The drawing under review shows one solid part. Ordinate dimensions are in mm from its lowest x, y, z. Round coordinates to 2 decimals unless told otherwise and drop trailing zeros. Write each loop counter-clockwise with the first axis right and the second up, starting at its lowest first coordinate (ties: lowest second). Pieces come first, ordered by that corner, then holes. Notation, with made-up numbers: (42.25, 70) -> (61.25, 70) arc R15 ccw to (61.25, 84) -> close; hole circle Ø4 at (73.5, 18.25). An arc over 180 degrees is marked (long way). Use CSV: the item, a comma, the result in double quotes. Start each with the question number.
1) Take a section at A-A, the plane z = 15. Give the boundary of the cut face in (x, y), then the cut area to 3 significant figures.
2) Take a section at D-D, the plane x = 72.5. Give the boundary of the cut face in (y, z).
3) For pin 1 Ø6 at (x, z) = (61.5, 8.5) entering from +Y; pin 2 Ø1.6 at (x, y) = (44.5, 27.5) entering from +Z; pin 3 Ø1 at (x, z) = (65.5, 13) entering from +Y, all flat-tipped, find the tip position at first contact; note any pin that passes through.
4) Take a section at B-B, the plane x = 6. Give the boundary of the cut face in (y, z).
5) Wall thickness on probe 1 along Y at (x, z) = (48, 15.25); probe 2 along Z at (x, y) = (33, 27.5); probe 3 along Y at (x, z) = (12, 12.5): over which ranges is each line inside the solid? List them lowest first. Write a range as [from, to].
6) Mouldability with a two-part tool opening along Z and no side actions: class the marked faces 1, 2 and 3 as released by +Z, released by -Z, zero draft, split by the parting line, or undercut.
7) Take a section at C-C, the plane y = 6.5. Give the boundary of the cut face in (x, z), then the cut area to 3 significant figures.
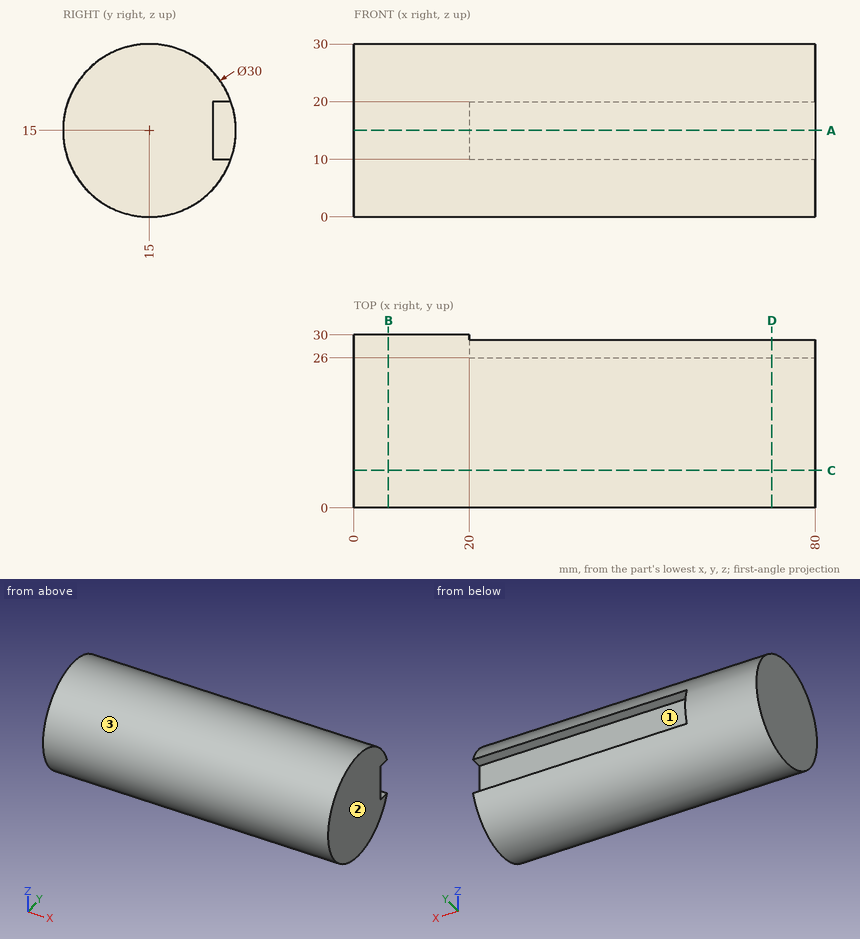
Values found:
1,outline,"(0, 0) -> (80, 0) -> (80, 26) -> (20, 26) -> (20, 30) -> (0, 30) -> close"
1,area,"2,160 mm²"
2,outline,"(26, 10) -> (26, 20) -> (29.14, 20) arc R15 ccw (long way) to (29.14, 10) -> close"
3,pin 1,"y = 29.14"
3,pin 2,"z = 24.39"
3,pin 3,"y = 26"
4,outline,"circle Ø30 at (15, 15)"
5,probe 1,"[0, 26]"
5,probe 2,"[6.71, 10], [20, 23.29]"
5,probe 3,"[0.21, 29.79]"
6,face 1,"undercut"
6,face 2,"zero draft"
6,face 3,"split by the parting line"
7,outline,"(0, 2.64) -> (80, 2.64) -> (80, 27.36) -> (0, 27.36) -> close"
7,area,"1,980 mm²"
